Read the model definition and answer for the solid it produces. Units are mm, in the model's axes. A direction names the side the tool comes from. Coordinates: 2 decimals unless noted, no trailing zeros. Order: outer loops, then holes, each group sorted by start corner. A loop starts at its lowest first (then second) coordinate and runs counter-clockwise, first axis right, second up.
```python
from build123d import *

# Parameters (mm, degrees)
CORTAR_EXTRUIR1_DEPTH = 2.9
REDONDEO1_R           = 10
CORTAR_EXTRUIR2_REACH = 39.094
CROQUIS3_R            = 1.75
CROQUIS4_R            = 2.75
CORTAR_EXTRUIR3_DEPTH = 18.1
CHAFL_N1_SIZE         = 1
CHAFL_N2_SIZE         = 0.5
CROQUIS5_R            = 13.05
CORTAR_EXTRUIR4_DEPTH = 4.9


with BuildPart() as part:
    # Croquis1 → Revolución1 (revolve)
    with BuildSketch(Plane.XY):
        Polygon((-16, 0), (-16, 4), (0, 4), (0, 20), (8, 20), (8, 0), align=None)
    revolve(axis=Axis((8, 0, 0), (-1, 0, 0)))

    # Croquis2 → Cortar-Extruir1 (cut)
    with BuildSketch(Plane(origin=(8, 0, 0), x_dir=(0, 0, -1), z_dir=(1, 0, 0))):
        with BuildLine():
            Line((-2.839199656, 15.194118815), (-7.049029232, 10.984289239))
            ThreePointArc((-7.049029232, 10.984289239), (-7.634375098, 9.528098398), (-6.988431485, 8.097756342))
            ThreePointArc((-6.988431485, 8.097756342), (-3.433318471, 0), (-6.988431485, -8.097756342))
            ThreePointArc((-6.988431485, -8.097756342), (-7.634375098, -9.528098398), (-7.049029232, -10.984289239))
            Line((-7.049029232, -10.984289239), (-2.839199656, -15.194118815))
            ThreePointArc((-2.839199656, -15.194118815), (-1.453779812, -15.779697972), (-0.052075025, -15.234248815))
            ThreePointArc((-0.052075025, -15.234248815), (6.516681529, 0), (-0.052075025, 15.234248815))
            ThreePointArc((-0.052075025, 15.234248815), (-1.453779812, 15.779697972), (-2.839199656, 15.194118815))
        make_face()
    extrude(amount=-CORTAR_EXTRUIR1_DEPTH, mode=Mode.SUBTRACT)

    # Redondeo1
    redondeo1_edges = [part.edges().sort_by_distance(p)[0] for p in [
        (0, -4, 0),
    ]]
    fillet(redondeo1_edges, radius=REDONDEO1_R)

    # Croquis3 → Cortar-Extruir2 (cut, up to next)
    with BuildSketch(Plane.ZY.offset(16), mode=Mode.PRIVATE) as cortar_extruir2_sk1:
        with Locations(Location((0, 0, 0), (0, 0, 270))):
            Circle(CROQUIS3_R)
    cortar_extruir2_tool1 = extrude(cortar_extruir2_sk1.sketch, amount=-CORTAR_EXTRUIR2_REACH, mode=Mode.PRIVATE) & part.part
    add(cortar_extruir2_tool1.solids().sort_by_distance((-16, 0, 0))[0], mode=Mode.SUBTRACT)

    # Croquis4 → Cortar-Extruir3 (cut)
    with BuildSketch(Plane(origin=(5.1, 0, 0), x_dir=(0, 0, -1), z_dir=(1, 0, 0))):
        with Locations(Location((0, 0, 0), (0, 0, 90))):
            Circle(CROQUIS4_R)
    extrude(amount=-CORTAR_EXTRUIR3_DEPTH, mode=Mode.SUBTRACT)

    # Chaflán1
    chafl_n1_edges = [part.edges().sort_by_distance(p)[0] for p in [
        (8, -20, 0),
    ]]
    chamfer(chafl_n1_edges, length=CHAFL_N1_SIZE)

    # Chaflán2
    chafl_n2_edges = [part.edges().sort_by_distance(p)[0] for p in [
        (8, -15.779697972, 1.453779812),
        (8, 0, -6.516681529),
        (8, 15.779697972, 1.453779812),
        (8, 13.089204027, 4.944114444),
        (8, 9.528098398, 7.634375098),
        (8, 0, 3.433318471),
        (8, -9.528098398, 7.634375098),
        (8, -13.089204027, 4.944114444),
    ]]
    chamfer(chafl_n2_edges, length=CHAFL_N2_SIZE)

    # Croquis5 → Cortar-Extruir4 (cut)
    with BuildSketch(Plane(origin=(8, 0, 0), x_dir=(0, 0, -1), z_dir=(1, 0, 0))):
        with Locations(Location((0, 0, 0), (0, 0, 80.792213194))):
            Circle(CROQUIS5_R)
    extrude(amount=-CORTAR_EXTRUIR4_DEPTH, mode=Mode.SUBTRACT)


solid = part.part
```
1) A cutting plane is placed at C-C, the plane x = -1. Determine the outline of the cut face in (y, z), and give its area (3 significant figures).
A:
outline: circle Ø19.28 at (0, 0); hole circle Ø5.5 at (0, 0)
area: 268 mm2
2) Which of the six approach directions +Z, -Z, +X, -X, +Y, -Y give full straight-line access (tool end or side, diameter ignored) to faces 1 (the cylindrical face through (5.584, -4.831, -12.123)), 2 (the cylindrical face through (-14.52, 0.38, -1.71)), 3 (the cylindrical face through (-12.958, -0.867, 3.905))?
A:
face 1: +X
face 2: +X, -X
face 3: -X
3) Determine the mould class of faces 4 (the cylindrical face through (3.549, -4.336, 19.524)), 5 (the flat face through (8, 4, -13)), 6 (the cylindrical face through (6.32, 15.78, 1.43)) for opening direction Y: pulls with the +Y half, pulls with the -Y half, needs draft (parallel to the pull), parting line crosses it, or undercut.
A:
face 4: parting line crosses it
face 5: needs draft
face 6: undercut
4) A cutting plane is placed at D-D, the plane x = -6.75. Determine the outline of the cut face in (y, z), and give its area (3 significant figures).
A:
outline: circle Ø9.09 at (0, 0); hole circle Ø5.5 at (0, 0)
area: 41.1 mm2
5) Straight lines are drawn through the part: line 1 (Y direction, x = 5.5, z = 0); line 2 (Z direction, x = 6.95, y = 0). For each, find the intervals that lie inside material, in ascending order.
A:
line 1: y = -20 to -15.18, 15.18 to 20
line 2: z = -20 to -13.05, 13.05 to 20
6) Flat-ended cylindrical pins translate along their axes: pin 1 Ø4 at (x, y) = (-1.5, -8) entering from +Z; pin 2 Ø4 at (y, z) = (0, 0) entering from +X; pin 3 Ø10 at (x, z) = (-9.5, -7.5) entering from -Y. Find the tip coordinate at first contact, or state that the pin passes through.
A:
pin 1: stops at z = 18.85
pin 2: stops at x = -13
pin 3: stops at y = -3.19
7) A cutting plane is placed at B-B, the plane y = 0. Determine the outline of the cut face in (x, z).
A:
outline: (-16, -4) - (-10, -4) arc R10 cw to (0, -14) - (0, -20) - (7, -20) - (8, -19) - (8, -13.05) - (3.1, -13.05) - (3.1, -2.75) - (-13, -2.75) - (-13, -1.75) - (-16, -1.75) - close; (-16, 1.75) - (-13, 1.75) - (-13, 2.75) - (3.1, 2.75) - (3.1, 13.05) - (8, 13.05) - (8, 19) - (7, 20) - (0, 20) - (0, 14) arc R10 cw to (-10, 4) - (-16, 4) - close
